Can you work these out from the model? Positions are in its coordinate system, mm. Give positions to 0.01 mm unless a question says otherwise; leave off trailing zeros. Order: outer loops, then holes, each group sorted by start corner. A loop starts at its lowest first (then second) coordinate and runs counter-clockwise, first axis right, second up. Notation, with made-up numbers: (77.25, 33.25) - (96.25, 33.25) arc R25 ccw to (96.25, 65.25) - close; hole circle Ø7 at (35, 82.5). An arc over 180 degrees is marked (long way). Use one line per item in the form item = value. Start each with the question number.
1) We'd pull the mould along Y, two halves only. Please class faces 1 (the cylindrical face through (-34.28, 28.498, 3.131)), 2 (the flat face through (-1, -30.45, 3)), 3 (the flat face through (-75.75, 0, 3)): released by +Y, released by -Y, zero draft, split by the parting line, or undercut.
2) Please list where these lines run through material, in increasing order: probe 1 along X at (y, z) = (27.5, 4.75); probe 2 along X at (y, z) = (-27, 3.5); probe 3 along Y at (x, z) = (-33.5, 4) (3 decimals).
3) For pin 1 (1.7 mm diameter, centred on x = -33.5, y = 27.275, fed in from +Z), with a flat end and sliding along its axis, tell me the tip position at first contact or that it passes through.
4) Suppose I cut it at A-A, the plane x = -20.75. Write out the boundary of the cut face in (y, z) (3 decimals), and give its area (3 significant figures).
```python
from build123d import *

# Parameters (mm, degrees)
SKETCH1_W              = 151.500000022
SKETCH1_H              = 60.9
BOSS_EXTRUDE1_DEPTH    = 6.35
M2_5_CLEARANCE_HOLE1_D = 2.9


with BuildPart() as part:
    # Sketch1 → Boss-Extrude1 (new body)
    with BuildSketch(Plane.XY):
        Rectangle(SKETCH1_W, SKETCH1_H)
    extrude(amount=BOSS_EXTRUDE1_DEPTH)

    # M2.5 Clearance Hole1 (through all)
    with Locations(Plane.XY.offset(6.35)):
        with Locations((-71.750000011, 27.275), (-59.000000011, 27.275), (-46.250000011, 27.275), (-33.500000011, 27.275), (-20.750000011, 27.275), (1.750001156, -27.275), (19.000000864, -27.275), (36.250000573, -27.275), (53.500000281, -27.275), (70.749999989, -27.275)):
            Hole(M2_5_CLEARANCE_HOLE1_D / 2)


solid = part.part
```
Result sheet:
q1.face_1 = undercut
q1.face_2 = released by -Y
q1.face_3 = zero draft
q2.probe_1 = -75.75 to -73.18, -70.32 to -60.43, -57.57 to -47.68, -44.82 to -34.93, -32.07 to -22.18, -19.32 to 75.75
q2.probe_2 = -75.75 to 0.33, 3.17 to 17.58, 20.42 to 34.83, 37.67 to 52.08, 54.92 to 69.33, 72.17 to 75.75
q2.probe_3 = -30.45 to 25.825, 28.725 to 30.45
q3.pin_1 = through
q4.outline = (-30.45, 0) - (25.825, 0) - (25.825, 6.35) - (-30.45, 6.35) - close; (28.725, 0) - (30.45, 0) - (30.45, 6.35) - (28.725, 6.35) - close
q4.area = 368 mm²
